```python
from build123d import *

# Parameters (mm, degrees)
SKETCH3_R           = 3
BOSS_EXTRUDE1_DEPTH = 3
SKETCH4_R           = 4
CUT_EXTRUDE1_DEPTH  = 3
SKETCH6_R           = 4
BOSS_EXTRUDE2_DEPTH = 25
SKETCH7_W           = 2.5
SKETCH7_H           = 1.19510496


with BuildPart() as part:
    # Sketch3 → Boss-Extrude1 (new, symmetric)
    with BuildSketch(Plane(origin=(0, 0, 0), x_dir=(1, 0, 0), z_dir=(0, 1, 0))):
        with BuildLine():
            Line((8.5, -6), (-8.5, -6))
            Line((-8.5, -6), (-8.5, 6))
            Line((-8.5, 6), (8.5, 6))
            ThreePointArc((8.5, 6), (14.5, 0), (8.5, -6))
        make_face()
        with Locations(Location((7, 0, 0), (0, 0, 270))):
            Circle(SKETCH3_R, mode=Mode.SUBTRACT)
    extrude(amount=BOSS_EXTRUDE1_DEPTH, both=True)

    # Sketch4 → Cut-Extrude1 (cut)
    with BuildSketch(Plane(origin=(0, 3, 0), x_dir=(1, 0, 0), z_dir=(0, 1, 0))):
        with Locations(Location((7, 0, 0), (0, 0, 270))):
            Circle(SKETCH4_R)
    extrude(amount=-CUT_EXTRUDE1_DEPTH, mode=Mode.SUBTRACT)

    # Sketch6 → Boss-Extrude2 (add, symmetric)
    with BuildSketch(Plane.XY):
        with Locations((-8.5, 0)):
            Circle(SKETCH6_R)
    extrude(amount=BOSS_EXTRUDE2_DEPTH, both=True)

    # Sketch7 → Cut-Revolve1 (revolve, cut)
    with BuildSketch(Plane(origin=(0, 0, 0), x_dir=(1, 0, 0), z_dir=(0, 1, 0))):
        with Locations((-4.5, 15)):
            Rectangle(SKETCH7_W, SKETCH7_H)
        with Locations((-4.5, -15)):
            Rectangle(SKETCH7_W, SKETCH7_H)
    revolve(axis=Axis((-8.5, 0, 25), (0, 0, -1)), mode=Mode.SUBTRACT)


solid = part.part
```
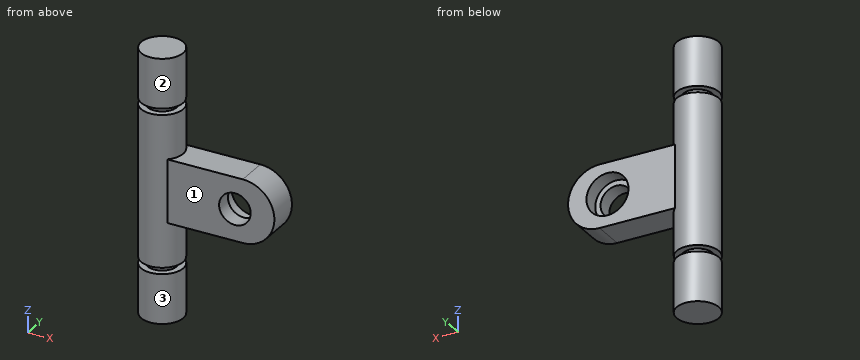
Check sheet for the modelled part. Datum: model origin and axes. Units: mm. Face numbers are marked on the shaded views. A direction names the side the tool comes from. Give positions to 0.01 mm unless a question says otherwise; leave off trailing zeros. Write each loop counter-clockwise with the first axis right and the second up, starting at its lowest first coordinate (ties: lowest second). Pieces come first, ordered by that corner, then holes. Notation, with made-up numbers: (-1, 85.25) -> (33, 85.25) arc R20 cw to (33, 113.25) -> close; hole circle Ø10 at (50.25, 34). An arc over 180 degrees is marked (long way). Use CSV: the item, a comma, the result in double quotes. Start each with the question number.
Q1. Cross-section at D-D on x = -3.5. Enter the section's corners in (y, z), and give its area (3 significant figures).
Q2. Cross-section at B-B on x = 7. Enter the section's corners in (y, z).
Q3. Cross-section at C-C on x = -7.5. Enter the section's corners in (y, z), and give its area (3 significant figures).
Q4. Cross-section at A-A on z = 0. Enter the section's corners in (x, y), and give its area (3 significant figures).
Q5. Depth check by flat-ended pin: P1, Ø7, axis at x = 7, z = 0, coming from the -Y side; P2, Ø1, axis at y = 2.5, z = -18.5, coming from the -X side; P3, Ø3, axis at x = -1.5, y = 0.5, coming from the +Z side. Enter the tip coordinate at first touch or a pass-through.
Q6. Tool access check on the marked faces 1, 2 and 3. Record the directions out of +Z, -Z, +X, -X, +Y, -Y that give a thin tool (end or side, any length) a straight path to the whole face; none if there is none.
Q7. Scan lines: line 1 along Z through (x, y) = (-11, 2.25); line 2 along Z through (x, y) = (7, -1.9); line 3 along Z through (x, y) = (6.75, 1.5). Record each from-to range of solid material in increasing order.
Working result:
1,outline,"(-3, -6) -> (3, -6) -> (3, 6) -> (-3, 6) -> close"
1,area,"72.0 mm^2"
2,outline,"(-3, -6) -> (3, -6) -> (3, -4) -> (0, -4) -> (0, -3) -> (-3, -3) -> close; (-3, 3) -> (0, 3) -> (0, 4) -> (3, 4) -> (3, 6) -> (-3, 6) -> close"
3,outline,"(-3.87, -25) -> (3.87, -25) -> (3.87, -15.6) -> (2.56, -15.6) -> (2.56, -14.4) -> (3.87, -14.4) -> (3.87, 14.4) -> (2.56, 14.4) -> (2.56, 15.6) -> (3.87, 15.6) -> (3.87, 25) -> (-3.87, 25) -> (-3.87, 15.6) -> (-2.56, 15.6) -> (-2.56, 14.4) -> (-3.87, 14.4) -> (-3.87, -14.4) -> (-2.56, -14.4) -> (-2.56, -15.6) -> (-3.87, -15.6) -> close"
3,area,"381 mm^2"
4,outline,"(-5.85, -3) -> (4, -3) -> (4, 0) -> (3, 0) -> (3, 3) -> (-5.85, 3) arc R4 ccw (long way) to start; (10, -3) -> (14.5, -3) -> (14.5, 3) -> (11, 3) -> (11, 0) -> (10, 0) -> close"
4,area,"125 mm^2"
5,P1,"stops at y = -3"
5,P2,"stops at x = -11.96"
5,P3,"stops at z = 6"
6,face 1,"+Z, -Z, +X, -Y"
6,face 2,"+Z"
6,face 3,"-Z"
7,line 1,"z = -25 to -15.6, -14.4 to 14.4, 15.6 to 25"
7,line 2,"z = -6 to -3, 3 to 6"
7,line 3,"z = -6 to -3.99, 3.99 to 6"
